Source: CAD feature listing. Evaluate the final solid. Frame: model axes, mm. A direction names the side the tool comes from. Give positions to 0.01 mm unless a question says otherwise; leave off trailing zeros. Loops run counter-clockwise (first coordinate to the right, second up) from the corner with the lowest first, then second, coordinate; pieces in that order, holes last.
Autodesk Inventor part; units mm, degrees
ref_plane "YZ Plane" through (0, 0, 0) normal (1, 0, 0) x (0, 1, 0)
ref_plane "XZ Plane" through (0, 0, 0) normal (0, 1, 0) x (-1, 0, 0)
ref_plane "XY Plane" through (0, 0, 0) normal (0, 0, 1) x (1, 0, 0)
sketch "草图1" plane through (0, 0, 0) normal (0, 0, 1) x (1, 0, 0)
  line L0 (11.5, -7.5) -> (-11.5, -7.5)
  line L1 (-11.5, -7.5) -> (-11.5, 7.5)
  line L2 (-11.5, 7.5) -> (11.5, 7.5)
  line L3 (11.5, 7.5) -> (11.5, -7.5)
  line L4 (11.5, -7.5) -> (-11.5, 7.5) construction
  line L5 (-11.5, -7.5) -> (11.5, 7.5) construction
  point P0 (0, 0)
  dimension "d0" = 23
  dimension "d1" = 15
extrude "拉伸1" add sketch "草图1" along normal blind 4
sketch "草图2" plane through (0, 0, 4) normal (0, 0, 1) x (1, 0, 0)
  circle A0 centre (0, 5) radius 1
  point P0 (0, 0)
  dimension "d4" = 2
  dimension "d10" = 5
extrude "拉伸2" cut sketch "草图2" against normal blind 4
sketch "草图3" plane through (0, 0, 0) normal (0, 0, -1) x (-1, 0, 0)
  line L0 (8.9655, -3.6241) -> (-8.9655, -3.6241)
  line L1 (-8.9655, -3.6241) -> (-8.9655, 3.6241)
  line L2 (-8.9655, 3.6241) -> (8.9655, 3.6241)
  line L3 (8.9655, 3.6241) -> (8.9655, -3.6241)
  line L4 (8.9655, -3.6241) -> (-8.9655, 3.6241) construction
  line L5 (-8.9655, -3.6241) -> (8.9655, 3.6241) construction
  point P0 (0, 0)
extrude "拉伸3" cut sketch "草图3" against normal blind 4
fillet "圆角1" radius 2 4 edges at (11.5, 7.5, 2) (-11.5, 7.5, 2) (-11.5, -7.5, 2) (11.5, -7.5, 2)
sketch "草图4" plane through (0, 0, 4) normal (0, 0, 1) x (1, 0, 0)
  circle A0 centre (0, 5) radius 1
  circle A1 centre (0, 5) radius 2
  point P0 (0, 0)
  dimension "d11" = 4
extrude "拉伸4" cut sketch "草图4" against normal blind 1.5 contours A0 | A1
fillet "圆角2" radius 2 2 edges at (1.4515, 3.6241, 3.25) (-1.4515, 3.6241, 3.25)
mirror "镜像1" about plane through (0, 0, 0) normal (0, 1, 0) of "拉伸4", "圆角2", "拉伸2"
properties part number "4mm隔热板"
(1) Section B-B, the plane z = 3.6. Return the cut outline in (x, y).
A:
outline: (-11.5, -5.5) arc R2 ccw to (-9.5, -7.5) - (9.5, -7.5) arc R2 ccw to (11.5, -5.5) - (11.5, 5.5) arc R2 ccw to (9.5, 7.5) - (-9.5, 7.5) arc R2 ccw to (-11.5, 5.5) - close; hole (-8.97, -3.62) - (-3.95, -3.62) arc R2 cw to (-1.98, -5.31) arc R2 ccw to (1.98, -5.31) arc R2 cw to (3.95, -3.62) - (8.97, -3.62) - (8.97, 3.62) - (3.95, 3.62) arc R2 cw to (1.98, 5.31) arc R2 ccw to (-1.98, 5.31) arc R2 cw to (-3.95, 3.62) - (-8.97, 3.62) - close
(2) Ray query, line 1 along Y through (x, z) = (0, 1.55); line 2 along X through (y, z) = (0.25, 3.55); line 3 along X through (y, z) = (-5, 0.95). Return the intervals inside material, ascending.
A:
line 1: y = -7.5 to -6, -4 to -3.62, 3.62 to 4, 6 to 7.5
line 2: x = -11.5 to -8.97, 8.97 to 11.5
line 3: x = -11.5 to -1, 1 to 11.5
(3) Section D-D, the plane x = 0. Return the cut outline in (y, z), then the cut area to 3 significant figures.
A:
outline: (-7.5, 0) - (-6, 0) - (-6, 2.5) - (-7, 2.5) - (-7, 4) - (-7.5, 4) - close; (-4, 0) - (-3.62, 0) - (-3.62, 2.5) - (-4, 2.5) - close; (3.62, 0) - (4, 0) - (4, 2.5) - (3.62, 2.5) - close; (6, 0) - (7.5, 0) - (7.5, 4) - (7, 4) - (7, 2.5) - (6, 2.5) - close
area: 10.9 mm2
(4) Mould query, pull axis Y, two halves, no side actions, for faces 1 (the flat face through (0, 3.624, 2)), 2 (the cylindrical face through (10.9, -6.93, 2.03)), 3 (the flat face through (-3, 5, 4)), 4 (the cylindrical face through (0, -4, 1)). Classes: pulls with the +Y half, pulls with the -Y half, needs draft (parallel to the pull), parting line crosses it, or undercut.
A:
face 1: undercut
face 2: pulls with the -Y half
face 3: needs draft
face 4: undercut
(5) Reachability of faces 5 (the flat face through (-1, 4, 2.5)), 6 (the flat face through (8.966, 0, 2)), 7 (the flat face through (-11.5, 0, 2)) from +Z, -Z, +X, -X, +Y, -Y: full face, straight path, thin tool, end or side. Return the list, or none.
A:
face 5: +Z
face 6: +Z, -Z
face 7: +Z, -Z, -X, +Y, -Y
(6) Section A-A, the plane x = -7.25. Return the cut outline in (y, z).
A:
outline: (-7.5, 0) - (-3.62, 0) - (-3.62, 4) - (-7.5, 4) - close; (3.62, 0) - (7.5, 0) - (7.5, 4) - (3.62, 4) - close
(7) Section C-C, the plane y = -0.5. Return the cut outline in (x, z).
A:
outline: (-11.5, 0) - (-8.97, 0) - (-8.97, 4) - (-11.5, 4) - close; (8.97, 0) - (11.5, 0) - (11.5, 4) - (8.97, 4) - close
(8) First-contact query: pin 1 (1 mm diameter, centred on x = 3, y = 4.5, fed in from -Z); pin 2 (2.5 mm diameter, centred on x = 0, y = -5, fed in from +Z). Flat tips, straight axial feed; report the tip coordinate or a pass-through.
A:
pin 1: stops at z = 0
pin 2: stops at z = 2.5
